Build history of the part. All positions in model axes, mm. A direction names the side the tool comes from. Coordinates: 2 decimals unless noted, no trailing zeros. Order: outer loops, then holes, each group sorted by start corner. A loop starts at its lowest first (then second) coordinate and runs counter-clockwise, first axis right, second up. Notation, with made-up numbers: (22, 16.25) - (52, 16.25) arc R14 cw to (52, 29.25) - close; hole circle Ø8 at (-25.5, 22). An arc over 180 degrees is marked (long way). Write each question's results on one line, items separated by ' | '.
Autodesk Inventor part; units mm, degrees
ref_plane "YZ Plane" through (0, 0, 0) normal (1, 0, 0) x (0, 1, 0)
ref_plane "XZ Plane" through (0, 0, 0) normal (0, 1, 0) x (-1, 0, 0)
ref_plane "XY Plane" through (0, 0, 0) normal (0, 0, 1) x (1, 0, 0)
sketch "Sketch1" plane through (0, 0, 0) normal (0, 0, 1) x (1, 0, 0)
  line L0 (-150, 125) -> (150, 125)
  line L1 (150, 125) -> (150, -125)
  line L2 (150, -125) -> (-150, -125)
  line L3 (-150, -125) -> (-150, 125)
  point P0 (0, 0)
  point P1 (0, 125)
  point P2 (150, 0)
  dimension "d0" = 300
  dimension "d1" = 250
extrude "Extrusion1" add sketch "Sketch1" along normal blind 40.35
sketch "Sketch2" plane through (0, 0, 40.35) normal (0, 0, 1) x (1, 0, 0)
  circle A0 centre (-120, 0) radius 5
  line L0 (150, 125) -> (-150, 125) construction
  line L1 (0, 125) -> (0, -125) construction
  line L2 (-150, -125) -> (150, -125) construction
  circle A1 centre (120, 0) radius 5
  point P0 (0, 0)
  dimension "d4" = 10
  dimension "d5" = 120
hole "Hole1" at (-120, 0, 40.35) at (120, 0, 40.35) direction (0, 0, -1) diameter 10 end through all counterbore diameter 20 counterbore depth 15
sketch "Sketch4" plane through (0, 0, 40.35) normal (0, 0, 1) x (1, 0, 0)
  circle A0 centre (-36, 11.5) radius 2
  line L0 (150, 125) -> (-150, 125) construction
  line L1 (0, 125) -> (0, -125) construction
  line L2 (-150, -125) -> (150, -125) construction
  line L3 (150, -125) -> (150, 125) construction
  line L4 (150, 0) -> (-150, 0) construction
  line L5 (-150, 125) -> (-150, -125) construction
  circle A1 centre (-36, -11.5) radius 2
  line L6 (0, -125) -> (0, 125) construction
  circle A2 centre (36, 11.5) radius 2
  circle A3 centre (36, -11.5) radius 2
  point P0 (0, 0)
  dimension "d13" = 4
  dimension "d14" = 11.5
  dimension "d15" = 36
hole "Hole2" at (-36, 11.5, 40.35) at (36, 11.5, 40.35) at (36, -11.5, 40.35) at (-36, -11.5, 40.35) direction (0, 0, -1) diameter 4 end through all counterbore diameter 12 counterbore depth 10
properties part number "base de madera grande"
1. Band-saw the part on B-B on x = 120. Give the cut face in (y, z).
Solved:
outline: (-125, 0) - (-5, 0) - (-5, 25.35) - (-10, 25.35) - (-10, 40.35) - (-125, 40.35) - close; (5, 0) - (125, 0) - (125, 40.35) - (10, 40.35) - (10, 25.35) - (5, 25.35) - close
2. Tool access for faces 1 (the face through (-30.677, 8.731, 35.28)), 2 (the face through (-2, 125, 20)): list every direction of +Z, -Z, +X, -X, +Y, -Y with a clear straight run to the whole face (end or side of a thin tool).
Solved:
face 1: +Z | face 2: +Z, -Z, +X, -X, +Y
3. Band-saw the part on A-A on y = 0. Give the cut face in (x, z), then the cut area to 3 significant figures.
Solved:
outline: (-150, 0) - (-125, 0) - (-125, 25.35) - (-130, 25.35) - (-130, 40.35) - (-150, 40.35) - close; (-115, 0) - (115, 0) - (115, 25.35) - (110, 25.35) - (110, 40.35) - (-110, 40.35) - (-110, 25.35) - (-115, 25.35) - close; (125, 0) - (150, 0) - (150, 40.35) - (130, 40.35) - (130, 25.35) - (125, 25.35) - close | area: 11,000 mm2
4. Probe line 1 (X direction, y = 0, z = 35.75); line 2 (X direction, y = 0, z = 12.5); line 3 (Y direction, x = -36, z = 9.5). List the from-to ranges inside material, lowest first.
Solved:
line 1: x = -150 to -130, -110 to 110, 130 to 150 | line 2: x = -150 to -125, -115 to 115, 125 to 150 | line 3: y = -125 to -13.5, -9.5 to 9.5, 13.5 to 125
5. Drop flat-ended pins along their axis: pin 1 Ø2.5 at (x, y) = (-36, -11.5) entering from +Z; pin 2 Ø3.5 at (x, y) = (33.5, 10) entering from +Z. Give the stop position or say it passes through.
Solved:
pin 1: passes through | pin 2: stops at z = 30.35
6. Two-plate mould, pull along X, no slides. Class faces 3 (the face through (2, -125, 20)), 4 (the face through (150, 2, 20)), 5 (the face through (115, -2, 25.35)): +X half, -X half, draft (parallel to the pull), parting line (faces both ways), or undercut.
Solved:
face 3: draft | face 4: +X half | face 5: undercut
